from build123d import *

# Parameters (mm, degrees)
EXTRUDE_2_DEPTH             = 6
EXTRUDE_3_DEPTH             = 6
SKETCH_4_R                  = 2.5
CUT_EXTRUDE_1_DEPTH         = 455.56865906
PATTERN_LINEAR_2_COUNT      = 2
PATTERN_LINEAR_2_PITCH      = 290.3
PATTERN_LINEAR_2_COUNT_DIR2 = 2
PATTERN_LINEAR_2_PITCH_DIR2 = 218
EXTRUDE_4_DEPTH             = 6
SKETCH_6_R                  = 2.25
CUT_EXTRUDE_2_DEPTH         = 455.766605854
SKETCH_7_R                  = 2.25
CUT_EXTRUDE_3_DEPTH         = 455.56865906


with BuildPart() as part:
    # Эскиз1 → Бобышка-Вытянуть2 (new body)
    with BuildSketch(Plane(origin=(0, 0, 0), x_dir=(1, 0, 0), z_dir=(0, 1, 0))):
        Polygon((50, -77.921508101), (50, -347.921508101), (-292.3, -347.921508101), (-292.3, -297.921508101), (0, -297.921508101), (0, -127.921508101), (-292.3, -127.921508101), (-292.3, -77.921508101), align=None)
    extrude(amount=EXTRUDE_2_DEPTH)

    # Эскиз2 → Бобышка-Вытянуть3 (add)
    with BuildSketch(Plane.XZ):
        Polygon((50, 315.921508101), (50, 109.921508101), (-292.3, 109.921508101), (-292.3, 121.921508101), (6, 121.921508101), (6, 303.921508101), (-292.3, 303.921508101), (-292.3, 315.921508101), align=None)
    extrude(amount=EXTRUDE_3_DEPTH)

    # Эскиз4 → Вырез-Вытянуть1 (cut, through all)
    with BuildSketch(Plane(origin=(0, 6, 0), x_dir=(1, 0, 0), z_dir=(0, 1, 0))):
        with Locations(Location((-266.3, -103.921508101, 0), (0, 0, 270))):
            Circle(SKETCH_4_R)
    cut_extrude_1 = extrude(amount=-CUT_EXTRUDE_1_DEPTH, mode=Mode.SUBTRACT)

    # Линейный массив2: Cut-Extrude 1 2 × 2
    with Locations(*[(i * PATTERN_LINEAR_2_PITCH, 0, j * PATTERN_LINEAR_2_PITCH_DIR2) for i in range(PATTERN_LINEAR_2_COUNT) for j in range(PATTERN_LINEAR_2_COUNT_DIR2) if (i, j) != (0, 0)]):
        add(cut_extrude_1, mode=Mode.SUBTRACT)

    # Эскиз5 → Бобышка-Вытянуть4 (add)
    with BuildSketch(Plane.XZ.offset(6)):
        Polygon((50, 315.921508101), (-292.3, 315.921508101), (-292.3, 262.921508101), (0, 262.921508101), (0, 162.921508101), (-292.3, 162.921508101), (-292.3, 109.921508101), (50, 109.921508101), align=None)
    extrude(amount=EXTRUDE_4_DEPTH)

    # Эскиз6 → Вырез-Вытянуть2 (cut, through all)
    with BuildSketch(Plane.XZ.offset(12)):
        with Locations(Location((14, 239.421508101, 0), (0, 0, 270))):
            Circle(SKETCH_6_R)
        with Locations(Location((40, 239.421508101, 0), (0, 0, 270))):
            Circle(SKETCH_6_R)
        with Locations(Location((40, 186.421508101, 0), (0, 0, 270))):
            Circle(SKETCH_6_R)
        with Locations(Location((14, 186.421508101, 0), (0, 0, 270))):
            Circle(SKETCH_6_R)
    extrude(amount=-CUT_EXTRUDE_2_DEPTH, mode=Mode.SUBTRACT)

    # Эскиз7 → Вырез-Вытянуть3 (cut, through all)
    with BuildSketch(Plane.XZ):
        with Locations(Location((-287.3, 342.921508101, 0), (0, 0, 270))):
            Circle(SKETCH_7_R)
        with Locations(Location((-287.3, 82.921508101, 0), (0, 0, 270))):
            Circle(SKETCH_7_R)
    extrude(amount=-CUT_EXTRUDE_3_DEPTH, mode=Mode.SUBTRACT)


solid = part.part
CAD build for the part. Positions are in the model's coordinates, mm. A direction names the side the tool comes from. Give positions to 0.01 mm unless a question says otherwise; leave off trailing zeros. Order: outer loops, then holes, each group sorted by start corner. A loop starts at its lowest first (then second) coordinate and runs counter-clockwise, first axis right, second up. Notation, with made-up numbers: (25, 17) - (78, 17) arc R7 ccw to (78, 24) - close; hole circle Ø6 at (-6, -26.5). An arc over 180 degrees is marked (long way). Answer in a Markdown table with one row per item.
1. Saw through at B-B, the plane z = 249. Give the cut face in (x, y).
Data:
| item | result |
|---|---|
| outline | (0, -12) - (50, -12) - (50, 6) - (0, 6) - (0, 0) - (6, 0) - (6, -6) - (0, -6) - close |
2. Pull direction Y, two halves, no side cores. Call faces 1 (the flat face through (-119, -6, 315.922)), 2 (the flat face through (-98, 0, 125)), 3 (the flat face through (-119, 6, 301)): pulls with the +Y half, pulls with the -Y half, needs draft (parallel to the pull), parting line crosses it, or undercut.
Data:
| item | result |
|---|---|
| face 1 | needs draft |
| face 2 | undercut |
| face 3 | pulls with the +Y half |
3. Tool access for faces 4 (the flat face through (-124, -6, 109.922)), 5 (the flat face through (-124, -12, 283)), 6 (the flat face through (-119, 0, 332)): list every direction of +Z, -Z, +X, -X, +Y, -Y with a clear straight run to the whole face (end or side of a thin tool).
Data:
| item | result |
|---|---|
| face 4 | -Z, +X, -X, -Y |
| face 5 | +Z, -Z, +X, -X, -Y |
| face 6 | +Z, +X, -X, -Y |
4. Flat gauge pins, fed straight in: pin 1 (6 mm diameter, centred on x = -266.3, z = 321.92, fed in from -Y); pin 2 (1.5 mm diameter, centred on x = -174.5, z = 136.5, fed in from +Y); pin 3 (2 mm diameter, centred on x = 11.5, y = -8.5, fed in from +Z). Where does each tip first touch, or does it go through?
Data:
| item | result |
|---|---|
| pin 1 | stops at y = 0 |
| pin 2 | stops at y = -6 |
| pin 3 | stops at z = 315.92 |
5. Saw through at A-A, the plane x = -110. Give the cut face in (y, z).
Data:
| item | result |
|---|---|
| outline | (-12, 109.92) - (0, 109.92) - (0, 77.92) - (6, 77.92) - (6, 127.92) - (0, 127.92) - (0, 121.92) - (-6, 121.92) - (-6, 162.92) - (-12, 162.92) - close; (-12, 262.92) - (-6, 262.92) - (-6, 303.92) - (0, 303.92) - (0, 297.92) - (6, 297.92) - (6, 347.92) - (0, 347.92) - (0, 315.92) - (-12, 315.92) - close |
6. Probe probe 1 along Z at (x, y) = (-287.3, 4.2); probe 2 along Z at (x, y) = (-37.5, 2); probe 3 along Z at (x, y) = (-254, -8.5). List the from-to ranges inside material, lowest first. Write a range as [from, to].
Data:
| item | result |
|---|---|
| probe 1 | z = [77.92, 80.67], [85.17, 127.92], [297.92, 340.67], [345.17, 347.92] |
| probe 2 | z = [77.92, 127.92], [297.92, 347.92] |
| probe 3 | z = [109.92, 162.92], [262.92, 315.92] |
